Work out the finished part from the listing and answer in its coordinate system (mm). A direction names the side the tool comes from. Give positions to 0.01 mm unless a question says otherwise; leave off trailing zeros. Order: outer loops, then holes, each group sorted by start corner. A loop starts at its lowest first (then second) coordinate and runs counter-clockwise, first axis right, second up.
```python
from build123d import *

# Parameters (mm, degrees)
SKETCH_1_W      = 70
SKETCH_1_H      = 30
SKETCH_1_R      = 1
EXTRUDE_1_DEPTH = 1.5
SKETCH_2_W      = 8
SKETCH_2_H      = 19
EXTRUDE_2_DEPTH = 4


with BuildPart() as part:
    # Эскиз1 → Бобышка-Вытянуть1 (new body)
    with BuildSketch(Plane(origin=(0, 0, 0), x_dir=(1, 0, 0), z_dir=(0, 1, 0))):
        Rectangle(SKETCH_1_W, SKETCH_1_H)
        with Locations(Location((-32.5, 12.5, 0), (0, 0, 270))):
            Circle(SKETCH_1_R, mode=Mode.SUBTRACT)
        with Locations(Location((32.5, 12.5, 0), (0, 0, 270))):
            Circle(SKETCH_1_R, mode=Mode.SUBTRACT)
        with Locations(Location((32.5, -12.5, 0), (0, 0, 270))):
            Circle(SKETCH_1_R, mode=Mode.SUBTRACT)
        with Locations(Location((-32.5, -12.5, 0), (0, 0, 270))):
            Circle(SKETCH_1_R, mode=Mode.SUBTRACT)
    extrude(amount=EXTRUDE_1_DEPTH)

    # Эскиз2 → Бобышка-Вытянуть2 (add)
    with BuildSketch(Plane(origin=(0, 1.5, 0), x_dir=(1, 0, 0), z_dir=(0, 1, 0))):
        with Locations((-25.5, 0)):
            Rectangle(SKETCH_2_W, SKETCH_2_H)
        with Locations((-12.5, 0)):
            Rectangle(SKETCH_2_W, SKETCH_2_H)
        with Locations((0.5, 0)):
            Rectangle(SKETCH_2_W, SKETCH_2_H)
    extrude(amount=EXTRUDE_2_DEPTH)


solid = part.part
```
1. The part is cut by section B-B (y = 2.7). Write down the section's boundary in (x, z).
Findings below:
outline: (-29.5, -9.5) - (-21.5, -9.5) - (-21.5, 9.5) - (-29.5, 9.5) - close; (-16.5, -9.5) - (-8.5, -9.5) - (-8.5, 9.5) - (-16.5, 9.5) - close; (-3.5, -9.5) - (4.5, -9.5) - (4.5, 9.5) - (-3.5, 9.5) - close
2. The part is cut by section A-A (x = -32.5). Write down the section's boundary in (y, z), then the cut area to 3 significant figures.
Findings below:
outline: (0, -15) - (1.5, -15) - (1.5, -13.5) - (0, -13.5) - close; (0, -11.5) - (1.5, -11.5) - (1.5, 11.5) - (0, 11.5) - close; (0, 13.5) - (1.5, 13.5) - (1.5, 15) - (0, 15) - close
area: 39.0 mm2
3. Given P1, Ø3, axis at y = 2.5, z = 7.5, coming from the -X side; P2, Ø3, axis at x = -12, y = 4, coming from the +Z side; P3, Ø3, axis at y = 4.5, z = -7.5, coming from the -X side; P4, Ø3, axis at y = 3.5, z = 1.5, coming from the +X side, each flat-ended and moving along its own axis, determine where each tip first touches the part or whether it passes through.
Findings below:
P1: stops at x = -35
P2: stops at z = 9.5
P3: stops at x = -29.5
P4: stops at x = 4.5
4. The part is cut by section D-D (x = 1). Write down the section's boundary in (y, z).
Findings below:
outline: (0, -15) - (1.5, -15) - (1.5, -9.5) - (5.5, -9.5) - (5.5, 9.5) - (1.5, 9.5) - (1.5, 15) - (0, 15) - close
5. Which of the six approach directions +Z, -Z, +X, -X, +Y, -Y give full straight-line access (tool end or side, diameter ignored) to faces 5 (the face through (-8.5, 3, 0)), 6 (the face through (-13, 3, 9.5)), 7 (the face through (-26, 3, -9.5)), 8 (the face through (0, 1, 15)), 9 (the face through (0, 5.5, 0))?
Findings below:
face 5: +Z, -Z, +Y
face 6: +Z, +X, -X, +Y
face 7: -Z, +X, -X, +Y
face 8: +Z, +X, -X, +Y, -Y
face 9: +Z, -Z, +X, -X, +Y
6. The mould has two halves that part along X. Classify faces 1 (the face through (-26, 5.5, 0)), 2 (the face through (-31.51, 0.74, -12.63)), 3 (the face through (-29.5, 3, 0)), 4 (the face through (4.5, 3, 0)): pulls with the +X half, pulls with the -X half, needs draft (parallel to the pull), parting line crosses it, or undercut.
Findings below:
face 1: needs draft
face 2: undercut
face 3: pulls with the -X half
face 4: pulls with the +X half
7. Straight lines are drawn through the part: probe 1 along X at (y, z) = (0.45, -12.5); probe 2 along X at (y, z) = (3.4, -6.75); probe 3 along Y at (x, z) = (24, 10.5). For each, find the intervals that lie inside material, in ascending order.
Findings below:
probe 1: x = -35 to -33.5, -31.5 to 31.5, 33.5 to 35
probe 2: x = -29.5 to -21.5, -16.5 to -8.5, -3.5 to 4.5
probe 3: y = 0 to 1.5
8. The part is cut by section C-C (z = -8.25). Write down the section's boundary in (x, y), then the cut area to 3 significant figures.
Findings below:
outline: (-35, 0) - (35, 0) - (35, 1.5) - (4.5, 1.5) - (4.5, 5.5) - (-3.5, 5.5) - (-3.5, 1.5) - (-8.5, 1.5) - (-8.5, 5.5) - (-16.5, 5.5) - (-16.5, 1.5) - (-21.5, 1.5) - (-21.5, 5.5) - (-29.5, 5.5) - (-29.5, 1.5) - (-35, 1.5) - close
area: 201 mm2
